Work out the finished part from the listing and answer in its coordinate system (mm). Give positions to 0.01 mm unless a question says otherwise; leave off trailing zeros. Loops run counter-clockwise (first coordinate to the right, second up) from the corner with the lowest first, then second, coordinate; pieces in that order, holes last. Notation, with made-up numbers: (19, 43.5) - (26, 43.5) arc R26 cw to (26, 60.5) - close; hole circle Ø8 at (16.5, 29.5). An arc over 180 degrees is marked (long way). One line per question, with ' | ' between items. Start each with the question number.
1. This flat-tipped pin is pushed along its axis until it touches: pin 1 (4.5 mm diameter, centred on x = 370, z = -55, fed in from +Y). Where does it stop, or does it pass through?
2. Find the intervals of material crossed by line 1 (X direction, y = 1.3, z = -305); line 2 (X direction, y = 3.1, z = -10); line 3 (Z direction, x = 130, y = 2.65), in increasing order.
3. Section A-A (x = 390.5) is taken. Determine the outline of the cut face in (y, z), plus the area to 3 significant figures.
4. Section B-B (y = 3.55) is taken. Give the number of separate pieces and of enclosed holes in the cut face, plus the area to 3 significant figures.
from build123d import *

# Parameters (mm, degrees)
ESQUISSE1_W             = 440
ESQUISSE1_H             = 360
ESQUISSE1_R             = 2.7
BOSS_EXTRU_1_DEPTH      = 5
ESQUISSE2_R             = 1.7
ESQUISSE2_R_2           = 2.5
ESQUISSE2_R_3           = 2.2
ESQUISSE2_W             = 66
ESQUISSE2_H             = 58
ESQUISSE2_W_2           = 50
ESQUISSE2_H_2           = 50
ENL_V_MAT_EXTRU_1_DEPTH = 6
CONG_1_R                = 10
ESQUISSE4_R             = 2.5
ESQUISSE4_W             = 30
ESQUISSE4_H             = 20
ENL_V_MAT_EXTRU_2_DEPTH = 10
CONG_2_R                = 6


with BuildPart() as part:
    # Esquisse1 → Boss.-Extru.1 (new body)
    with BuildSketch(Plane(origin=(0, 0, 0), x_dir=(1, 0, 0), z_dir=(0, 1, 0))):
        with Locations((220, 180)):
            Rectangle(ESQUISSE1_W, ESQUISSE1_H)
        with Locations((40, 350)):
            Circle(ESQUISSE1_R, mode=Mode.SUBTRACT)
        with Locations((130, 350)):
            Circle(ESQUISSE1_R, mode=Mode.SUBTRACT)
        with Locations((220, 350)):
            Circle(ESQUISSE1_R, mode=Mode.SUBTRACT)
        with Locations((310, 350)):
            Circle(ESQUISSE1_R, mode=Mode.SUBTRACT)
        with Locations((400, 350)):
            Circle(ESQUISSE1_R, mode=Mode.SUBTRACT)
        with Locations((400, 10)):
            Circle(ESQUISSE1_R, mode=Mode.SUBTRACT)
        with Locations((310, 10)):
            Circle(ESQUISSE1_R, mode=Mode.SUBTRACT)
        with Locations((220, 10)):
            Circle(ESQUISSE1_R, mode=Mode.SUBTRACT)
        with Locations((130, 10)):
            Circle(ESQUISSE1_R, mode=Mode.SUBTRACT)
        with Locations((40, 10)):
            Circle(ESQUISSE1_R, mode=Mode.SUBTRACT)
        with Locations((10, 217.36725867)):
            Circle(ESQUISSE1_R, mode=Mode.SUBTRACT)
        with Locations((10, 317.36725867)):
            Circle(ESQUISSE1_R, mode=Mode.SUBTRACT)
        with Locations((10, 42.63274133)):
            Circle(ESQUISSE1_R, mode=Mode.SUBTRACT)
        with Locations((10, 142.63274133)):
            Circle(ESQUISSE1_R, mode=Mode.SUBTRACT)
        with Locations((430, 142.63274133)):
            Circle(ESQUISSE1_R, mode=Mode.SUBTRACT)
        with Locations((430, 42.63274133)):
            Circle(ESQUISSE1_R, mode=Mode.SUBTRACT)
        with Locations((430, 317.36725867)):
            Circle(ESQUISSE1_R, mode=Mode.SUBTRACT)
        with Locations((430, 217.36725867)):
            Circle(ESQUISSE1_R, mode=Mode.SUBTRACT)
    extrude(amount=BOSS_EXTRU_1_DEPTH)

    # Esquisse2 → Enlèv. mat.-Extru.1 (cut, through all)
    with BuildSketch(Plane(origin=(0, 5, 0), x_dir=(1, 0, 0), z_dir=(0, 1, 0))):
        with Locations((30, 200)):
            Circle(ESQUISSE2_R)
        with Locations((70, 200)):
            Circle(ESQUISSE2_R)
        with Locations((70, 160)):
            Circle(ESQUISSE2_R)
        with Locations((30, 160)):
            Circle(ESQUISSE2_R)
        with Locations((222.5, 217.5)):
            Circle(ESQUISSE2_R_2)
        with Locations((297.5, 217.5)):
            Circle(ESQUISSE2_R_2)
        with Locations((222.5, 142.5)):
            Circle(ESQUISSE2_R_2)
        with Locations((297.5, 142.5)):
            Circle(ESQUISSE2_R_2)
        with Locations((407, 142.5)):
            Circle(ESQUISSE2_R_3)
        with Locations((357, 142.5)):
            Circle(ESQUISSE2_R_3)
        with Locations((357, 217.5)):
            Circle(ESQUISSE2_R_3)
        with Locations((407, 217.5)):
            Circle(ESQUISSE2_R_3)
        with Locations((163, 142.5)):
            Circle(ESQUISSE2_R_3)
        with Locations((113, 142.5)):
            Circle(ESQUISSE2_R_3)
        with Locations((113, 217.5)):
            Circle(ESQUISSE2_R_3)
        with Locations((163, 217.5)):
            Circle(ESQUISSE2_R_3)
        with Locations((138, 180)):
            Rectangle(ESQUISSE2_W, ESQUISSE2_H)
        with Locations((382, 180)):
            Rectangle(ESQUISSE2_W, ESQUISSE2_H)
        with Locations((260, 180)):
            Rectangle(ESQUISSE2_W_2, ESQUISSE2_H_2)
        with BuildLine():
            ThreePointArc((215.25, 181.089724736), (210.5, 180), (215.25, 178.910275264))
            ThreePointArc((215.25, 178.910275264), (220, 180), (215.25, 181.089724736))
        make_face()
        with BuildLine():
            ThreePointArc((304.75, 178.910275264), (309.5, 180), (304.75, 181.089724736))
            ThreePointArc((304.75, 181.089724736), (300, 180), (304.75, 178.910275264))
        make_face()
    extrude(amount=-ENL_V_MAT_EXTRU_1_DEPTH, mode=Mode.SUBTRACT)

    # Congé1
    cong_1_edges = [part.edges().sort_by_distance(p)[0] for p in [
        (415, 2.5, -209),
        (415, 2.5, -151),
        (349, 2.5, -151),
        (349, 2.5, -209),
        (105, 2.5, -151),
        (105, 2.5, -209),
        (171, 2.5, -209),
        (171, 2.5, -151),
        (285, 2.5, -205),
        (285, 2.5, -155),
        (235, 2.5, -155),
        (235, 2.5, -205),
    ]]
    fillet(cong_1_edges, radius=CONG_1_R)

    # Esquisse4 → Enlèv. mat.-Extru.2 (cut)
    with BuildSketch(Plane(origin=(0, 5, 0), x_dir=(1, 0, 0), z_dir=(0, 1, 0))):
        with Locations((70, 290)):
            Circle(ESQUISSE4_R)
        with Locations((120, 290)):
            Circle(ESQUISSE4_R)
        with Locations((70, 305)):
            Circle(ESQUISSE4_R)
        with Locations((70, 275)):
            Circle(ESQUISSE4_R)
        with Locations((120, 275)):
            Circle(ESQUISSE4_R)
        with Locations((120, 305)):
            Circle(ESQUISSE4_R)
        with Locations((320, 305)):
            Circle(ESQUISSE4_R)
        with Locations((320, 275)):
            Circle(ESQUISSE4_R)
        with Locations((370, 275)):
            Circle(ESQUISSE4_R)
        with Locations((370, 305)):
            Circle(ESQUISSE4_R)
        with Locations((320, 290)):
            Circle(ESQUISSE4_R)
        with Locations((370, 290)):
            Circle(ESQUISSE4_R)
        with Locations((370, 70)):
            Circle(ESQUISSE4_R)
        with Locations((320, 70)):
            Circle(ESQUISSE4_R)
        with Locations((370, 55)):
            Circle(ESQUISSE4_R)
        with Locations((370, 85)):
            Circle(ESQUISSE4_R)
        with Locations((320, 85)):
            Circle(ESQUISSE4_R)
        with Locations((320, 55)):
            Circle(ESQUISSE4_R)
        with Locations((120, 55)):
            Circle(ESQUISSE4_R)
        with Locations((120, 85)):
            Circle(ESQUISSE4_R)
        with Locations((70, 85)):
            Circle(ESQUISSE4_R)
        with Locations((70, 55)):
            Circle(ESQUISSE4_R)
        with Locations((120, 70)):
            Circle(ESQUISSE4_R)
        with Locations((70, 70)):
            Circle(ESQUISSE4_R)
        with Locations((95, 290)):
            Rectangle(ESQUISSE4_W, ESQUISSE4_H)
        with Locations((345, 290)):
            Rectangle(ESQUISSE4_W, ESQUISSE4_H)
        with Locations((345, 70)):
            Rectangle(ESQUISSE4_W, ESQUISSE4_H)
        with Locations((95, 70)):
            Rectangle(ESQUISSE4_W, ESQUISSE4_H)
    extrude(amount=-ENL_V_MAT_EXTRU_2_DEPTH, mode=Mode.SUBTRACT)

    # Congé2
    cong_2_edges = [part.edges().sort_by_distance(p)[0] for p in [
        (80, 2.5, -60),
        (80, 2.5, -80),
        (110, 2.5, -80),
        (110, 2.5, -60),
        (360, 2.5, -80),
        (360, 2.5, -60),
        (330, 2.5, -60),
        (330, 2.5, -80),
        (110, 2.5, -300),
        (110, 2.5, -280),
        (80, 2.5, -280),
        (80, 2.5, -300),
        (360, 2.5, -300),
        (360, 2.5, -280),
        (330, 2.5, -280),
        (330, 2.5, -300),
    ]]
    fillet(cong_2_edges, radius=CONG_2_R)


solid = part.part
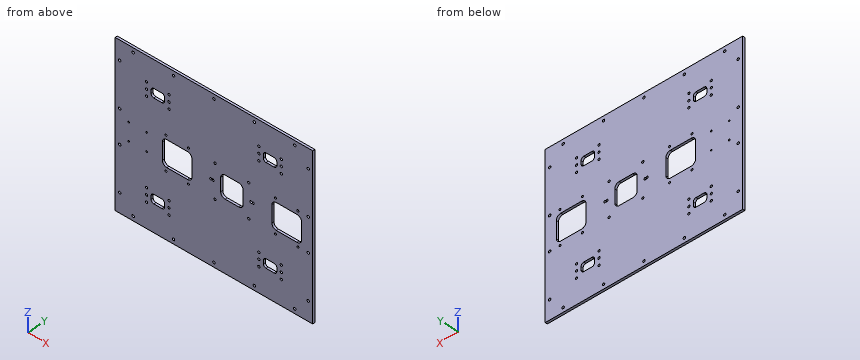
Conclusion:
1) pin 1: through
2) line 1: 0 to 67.5, 72.5 to 117.5, 122.5 to 317.5, 322.5 to 367.5, 372.5 to 440 | line 2: 0 to 37.3, 42.7 to 127.3, 132.7 to 217.3, 222.7 to 307.3, 312.7 to 397.3, 402.7 to 440 | line 3: -360 to -352.7, -347.3 to -209, -151 to -12.7, -7.3 to 0
3) outline: (0, -360) - (5, -360) - (5, -209) - (0, -209) - close; (0, -151) - (5, -151) - (5, 0) - (0, 0) - close | area: 1,510 mm²
4) separate pieces: 1 | enclosed holes: 67 | area: 145,000 mm²
